Check sheet for the modelled part. Datum: model origin and axes. Units: mm. Face numbers are marked on the shaded views. A direction names the side the tool comes from. Round coordinates to 2 decimals unless told otherwise and drop trailing zeros. Loops run counter-clockwise (first coordinate to the right, second up) from the corner with the lowest first, then second, coordinate; pieces in that order, holes last. Notation, with made-up numbers: (22.25, 41) - (70.25, 41) arc R22 ccw to (70.25, 58) - close; hole circle Ø1 at (82, 71.25). An arc over 180 degrees is marked (long way). Return JSON: item names as keys, results as strings.
from build123d import *

# Parameters (mm, degrees)
SKETCH2_W                = 30
SKETCH2_H                = 14
SKETCH2_R                = 3
BOSS_EXTRUDE1_DEPTH      = 10
SKETCH2_5_R              = 3
CUT_EXTRUDE1_DEPTH       = 3
BOSS_EXTRUDE2_DEPTH      = 40
BOSS_EXTRUDE2_DEPTH_BACK = 20
SKETCH3_W                = 30
SKETCH3_H                = 20
SKETCH3_R                = 6
BOSS_EXTRUDE3_DEPTH      = 10
CUT_EXTRUDE2_START       = -7
CUT_EXTRUDE2_DEPTH       = 7


with BuildPart() as part:
    # Sketch2 → Boss-Extrude1 (new body)
    # profile 1 of 3: a face of its own
    with BuildSketch(Plane(origin=(0, 0, 0), x_dir=(0, 1, 0), z_dir=(0, 0, 1))):
        with BuildLine():
            ThreePointArc((0, -16), (-13.330167524, -8.849103559), (-14.745004109, 6.211670776))
            Line((-14.745004109, 6.211670776), (-30, -30))
            Line((-30, -30), (-30, -40))
            Line((-30, -40), (0, -40))
            Line((0, -40), (0, -16))
        make_face()
    # profile 2 of 3: a face of its own
    with BuildSketch(Plane(origin=(0, 0, 0), x_dir=(0, 1, 0), z_dir=(0, 0, 1))):
        with Locations((-15, -63)):
            Rectangle(SKETCH2_W, SKETCH2_H)
    # profile 3 of 3: a face of its own
    with BuildSketch(Plane(origin=(0, 0, 0), x_dir=(0, 1, 0), z_dir=(0, 0, 1))):
        with BuildLine():
            Line((0, -40), (-30, -40))
            Line((-30, -40), (-30, -56))
            Line((-30, -56), (0, -56))
            Line((0, -56), (0, -51))
            ThreePointArc((0, -51), (-3, -48), (0, -45))
            Line((0, -45), (0, -40))
        make_face()
        with Locations(Location((-20, -48, 0), (0, 0, 270))):
            Circle(SKETCH2_R, mode=Mode.SUBTRACT)
    extrude(amount=-BOSS_EXTRUDE1_DEPTH)

    # Sketch2_5 → Cut-Extrude1 (cut)
    with BuildSketch(Plane(origin=(0, 0, 0), x_dir=(0, 1, 0), z_dir=(0, 0, 1))):
        with BuildLine():
            Line((0, -40), (-30, -40))
            Line((-30, -40), (-30, -56))
            Line((-30, -56), (0, -56))
            Line((0, -56), (0, -51))
            ThreePointArc((0, -51), (-3, -48), (0, -45))
            Line((0, -45), (0, -40))
        make_face()
        with Locations(Location((-20, -48, 0), (0, 0, 270))):
            Circle(SKETCH2_5_R, mode=Mode.SUBTRACT)
    extrude(amount=-CUT_EXTRUDE1_DEPTH, mode=Mode.SUBTRACT)

    # Sketch2_6 → Boss-Extrude2 (add, two sides: drawn at the far end of the back side and taken through both)
    with BuildSketch(Plane(origin=(0, 0, 0), x_dir=(0, 1, 0), z_dir=(0, 0, 1)).offset(-BOSS_EXTRUDE2_DEPTH_BACK)):
        with BuildLine():
            ThreePointArc((0, 16), (-8.849103559, 13.330167524), (-14.745004109, 6.211670776))
            ThreePointArc((-14.745004109, 6.211670776), (-13.330167524, -8.849103559), (0, -16))
            Line((0, -16), (0, -11))
            ThreePointArc((0, -11), (-10.895252583, -1.514421063), (-3, 10.583005244))
            Line((-3, 10.583005244), (-3, 14))
            Line((-3, 14), (0, 14))
            Line((0, 14), (0, 16))
        make_face()
    extrude(amount=BOSS_EXTRUDE2_DEPTH + BOSS_EXTRUDE2_DEPTH_BACK)

    # Sketch3 → Boss-Extrude3 (add)
    with BuildSketch(Plane.YZ.offset(70)):
        with Locations((-15, -20)):
            Rectangle(SKETCH3_W, SKETCH3_H)
        with Locations(Location((-15, -20, 0), (0, 0, 270))):
            Circle(SKETCH3_R, mode=Mode.SUBTRACT)
    extrude(amount=-BOSS_EXTRUDE3_DEPTH)

    # Mirror1: part across face


with BuildPart() as part_1:
    add(part.part)
    add(part.part.mirror(Plane(origin=(21.317391304, 0, 2.734782609), x_dir=(0, 0, 1), z_dir=(0, 1, 0))))

    # Sketch4 → Cut-Extrude2 (cut)
    with BuildSketch(Plane.XY.offset(40).offset(CUT_EXTRUDE2_START)):
        with BuildLine():
            ThreePointArc((3, -10.583005244), (1.514421063, -10.895252583), (0, -11))
            Line((0, -11), (0, -16))
            ThreePointArc((0, -16), (1.506695336, -15.928900438), (3, -15.716233646))
            Line((3, -15.716233646), (3, -10.583005244))
        make_face()
        with BuildLine():
            Line((0, -16), (0, -11))
            ThreePointArc((0, -11), (-1.514421063, -10.895252583), (-3, -10.583005244))
            Line((-3, -10.583005244), (-3, -15.716233646))
            ThreePointArc((-3, -15.716233646), (-1.506695336, -15.928900438), (0, -16))
        make_face()
    extrude(amount=CUT_EXTRUDE2_DEPTH, mode=Mode.SUBTRACT)


solid = part_1.part
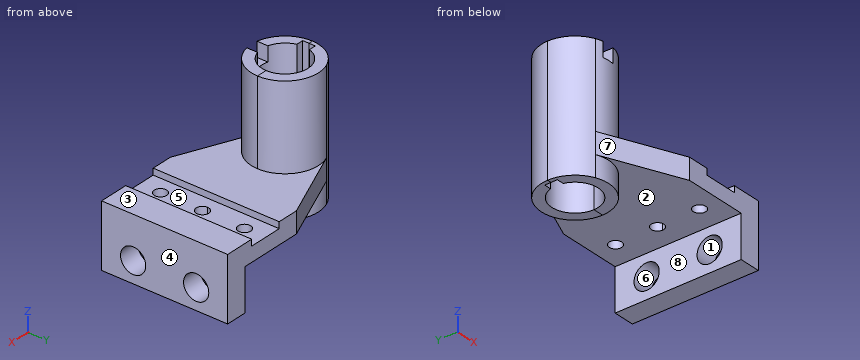
Q1. Sectioned sample at B-B (z = -6). Enter the section's corners in (x, y) (3 decimals).
Answer key:
{"outline": "(-6.212, -14.745) - (30, -30) - (70, -30) - (70, 30) - (30, 30) - (-6.212, 14.745) arc R16 ccw to start; hole (-14, -3) - (-10.583, -3) arc R11 ccw (long way) to (-10.583, 3) - (-14, 3) - close; hole circle Ø6 at (48, -20); hole circle Ø6 at (48, 0); hole circle Ø6 at (48, 20)"}
Q2. Sectioned sample at C-C (y = -4.5). Enter the section's corners in (x, z), plus the area to 3 significant figures.
Answer key:
{"outline": "(-15.35, -20) - (-10.04, -20) - (-10.04, 40) - (-15.35, 40) - close; (10.04, -20) - (15.35, -20) - (15.35, -10) - (60, -10) - (60, -30) - (70, -30) - (70, 0) - (56, 0) - (56, -3) - (40, -3) - (40, 0) - (15.35, 0) - (15.35, 40) - (10.04, 40) - close", "area": "1,340 mm²"}
Q3. Sectioned sample at A-A (x = 48). Enter the section's corners in (y, z), plus the area to 3 significant figures.
Answer key:
{"outline": "(-30, -10) - (-23, -10) - (-23, -3) - (-30, -3) - close; (-17, -10) - (-3, -10) - (-3, -3) - (-17, -3) - close; (3, -10) - (17, -10) - (17, -3) - (3, -3) - close; (23, -10) - (30, -10) - (30, -3) - (23, -3) - close", "area": "294 mm²"}
Q4. Draft check along Z on the marked faces 1, 2, 3 and 4. Enter one of: released by +Z, released by -Z, zero draft, split by the parting line, or undercut.
Answer key:
{"face 1": "undercut", "face 2": "released by -Z", "face 3": "released by +Z", "face 4": "zero draft"}
Q5. Depth check by flat-ended pin: P1, Ø12, axis at x = 48, y = 16, coming from the +Z side; P2, Ø15.5, axis at y = -15, z = -20, coming from the -X side; P3, Ø3.5, axis at y = -2, z = 20.5, coming from the +X side; P4, Ø5.5, axis at x = 48, y = -20, coming from the +Z side. Enter the tip coordinate at first touch or a pass-through.
Answer key:
{"P1": "stops at z = -3", "P2": "stops at x = -14.26", "P3": "stops at x = 16", "P4": "passes through"}
Q6. Tool access check on the marked faces 5, 6, 7 and 8. Record the directions out of +Z, -Z, +X, -X, +Y, -Y that give a thin tool (end or side, any length) a straight path to the whole face; none if there is none.
Answer key:
{"face 5": "+Z, +Y, -Y", "face 6": "+X", "face 7": "+Z, -Z, -X, -Y", "face 8": "-Z, +Y, -Y"}
Q7. Scan lines: probe 1 along Y at (x, z) = (65, -20); probe 2 along Y at (x, z) = (-13, -4); probe 3 along X at (y, z) = (20, -7). Record each from-to range of solid material in increasing order. Write a range as [from, to].
Answer key:
{"probe 1": "y = [-30, -21], [-9, 9], [21, 30]", "probe 2": "y = [-9.33, -3], [3, 9.33]", "probe 3": "x = [6.26, 45], [51, 70]"}
Q8. Sectioned sample at D-D (z = 9.5). Enter the section's corners in (x, y) (3 decimals), plus the area to 3 significant figures.
Answer key:
{"outline": "circle Ø32 at (0, 0); hole (-14, -3) - (-10.583, -3) arc R11 ccw (long way) to (-10.583, 3) - (-14, 3) - close", "area": "405 mm²"}
